Can you work these out from the model? Positions are in its coordinate system, mm. A direction names the side the tool comes from. Give positions to 0.01 mm unless a question says otherwise; leave off trailing zeros. Write each loop counter-clockwise with the first axis right and the second up, starting at its lowest first coordinate (ties: lowest second). Pieces come first, ordered by that corner, then holes. Notation, with made-up numbers: (44.5, -26) -> (97.5, -26) arc R17 cw to (97.5, -12) -> close; hole circle Ø7 at (-21, 68). An arc over 180 degrees is marked (long way). One line per item, written item: value.
from build123d import *
from build123d.topology import SkipClean

# Parameters (mm, degrees)
SKETCH1_R           = 4
BOSS_EXTRUDE1_DEPTH = 39.85
BOSS_EXTRUDE2_START = 5
BOSS_EXTRUDE2_DEPTH = 5
CUT_EXTRUDE1_START  = -5
CUT_EXTRUDE1_DEPTH  = 5


with BuildPart() as part:
    # Sketch1 → Boss-Extrude1 (new body)
    with BuildSketch(Plane.XY):
        Circle(SKETCH1_R)
    extrude(amount=-BOSS_EXTRUDE1_DEPTH)

    # Sketch2 → Boss-Extrude2 (add)
    with SkipClean():  # the faces are left unmerged after this step: merging them gives an invalid solid
        with BuildSketch(Plane.XY.offset(BOSS_EXTRUDE2_START)):
            with BuildLine():
                Line((-2, 3.464101615), (-2, -3.464101615))
                ThreePointArc((-2, -3.464101615), (-4, 0), (-2, 3.464101615))
            make_face()
            with BuildLine():
                Line((2, 3.464101615), (2, -3.464101615))
                ThreePointArc((2, -3.464101615), (4, 0), (2, 3.464101615))
            make_face()
        extrude(amount=-BOSS_EXTRUDE2_DEPTH)

    # Sketch3 → Cut-Extrude1 (cut)
    with SkipClean():  # the faces are left unmerged after this step: merging them gives an invalid solid
        with BuildSketch(Plane(origin=(0, 0, -39.85), x_dir=(-1, 0, 0), z_dir=(0, 0, -1)).offset(CUT_EXTRUDE1_START)):
            with BuildLine():
                Line((-1.925, 3.506333555), (-1.925, -3.506333555))
                ThreePointArc((-1.925, -3.506333555), (-4, 0), (-1.925, 3.506333555))
            make_face()
            with BuildLine():
                Line((1.925, 3.506333555), (1.925, -3.506333555))
                ThreePointArc((1.925, -3.506333555), (4, 0), (1.925, 3.506333555))
            make_face()
        extrude(amount=CUT_EXTRUDE1_DEPTH, mode=Mode.SUBTRACT)


solid = part.part
1) I need wall thicknesses on L1, parallel to Z at x = -2.5, y = -0.5; L2, parallel to Z at x = -0.5, y = 0; L3, parallel to Y at x = 2, z = -6. Which ranges of each line are inside material? Lowest first, please.
Answer list:
L1: z = -34.85 to 5
L2: z = -39.85 to 0
L3: y = -3.46 to 3.46
2) If we section it at A-A (y = 0): Write out the boundary of the cut face in (x, z) (3 decimals), and give its area (3 significant figures).
Answer list:
outline: (-4, -34.85) -> (-1.925, -34.85) -> (-1.925, -39.85) -> (1.925, -39.85) -> (1.925, -34.85) -> (4, -34.85) -> (4, 5) -> (2, 5) -> (2, 0) -> (-2, 0) -> (-2, 5) -> (-4, 5) -> close
area: 318 mm^2
3) For faces 1 (the face through (-3, 0, 5)), 2 (the face through (0, 0, 0)), 3 (the face through (0, 0, -39.85)), 4 (the face through (1.925, 0, -37)), 5 (the face through (-1.925, 0, -37)), which set-ups out of +Z, -Z, +X, -X, +Y, -Y let a thin tool reach every point of the face, with its end or its side?
Answer list:
face 1: +Z, +X, -X, +Y, -Y
face 2: +Z, +Y, -Y
face 3: -Z, +X, -X, +Y, -Y
face 4: -Z, +X, +Y, -Y
face 5: -Z, -X, +Y, -Y
4) If we section it at C-C (z = -30): Write out the boundary of the cut face in (x, y).
Answer list:
outline: circle Ø8 at (0, 0)
5) If we section it at B-B (x = 2.5): Write out the boundary of the cut face in (y, z), and give its area (3 significant figures).
Answer list:
outline: (-3.12, -34.85) -> (3.12, -34.85) -> (3.12, 5) -> (-3.12, 5) -> close
area: 249 mm^2
6) If we section it at D-D (x = 0): Write out the boundary of the cut face in (y, z).
Answer list:
outline: (-4, -39.85) -> (4, -39.85) -> (4, 0) -> (-4, 0) -> close
7) Will these pins go through, and if not, where does the flat tip stop? pin 1 (2.5 mm diameter, centred on y = -1, z = -37, fed in from -X) (3 decimals); pin 2 (1 mm diameter, centred on y = -1.5, z = -22.5, fed in from +X); pin 3 (0.6 mm diameter, centred on x = -3, y = 1.5, fed in from -Z).
Answer list:
pin 1: stops at x = -1.925
pin 2: stops at x = 3.87
pin 3: stops at z = -34.85
